Part model, mm, in its own coordinate system. Face numbers are marked on the shaded views. A direction names the side the tool comes from. Coordinates: 2 decimals unless noted, no trailing zeros. Write each loop counter-clockwise with the first axis right and the second up, starting at its lowest first coordinate (ties: lowest second). Pieces come first, ordered by that corner, then holes. Notation, with made-up numbers: (-9.75, 72.25) -> (27.25, 72.25) arc R15 cw to (27.25, 99.25) -> close; hole circle Ø5 at (7.25, -38.5). An arc over 180 degrees is marked (long way). One line per question, with ' | ' between items. Start each with the question number.
Item 1: Saw through at C-C (y = 12.5). List the corners of the cut face in (x, z).
Item 2: Probe probe 1 along Y at (x, z) = (0, 6.25); probe 2 along Y at (x, z) = (0.5, 2); probe 3 along X at (y, z) = (1, 11.5). List the from-to ranges inside material, lowest first. Write a range as [from, to].
Item 3: Saw through at A-A (x = 0). List the corners of the cut face in (y, z), and give its area (3 significant figures).
Item 4: Two-plate mould, pull along Y, no slides. Class the marked faces 1 and 2: pulls with the +Y half, pulls with the -Y half, needs draft (parallel to the pull), parting line crosses it, or undercut.
Item 5: Saw through at B-B (z = 6). Count the separate pieces of the cut face and the enclosed holes in it, and give its area (3 significant figures).
Item 6: 3-axis set-ups, long thin cutter, end or side, ignore diameter. For the marked faces 3 and 4: which of +Z, -Z, +X, -X, +Y, -Y reach the whole face in a straight line?
Item 7: Pin check, flat tips, straight feed: pin 1 (5 mm diameter, centred on x = 9.5, z = 2.5, fed in from -Y); pin 2 (13 mm diameter, centred on x = -40.7, y = 23.5, fed in from -Z); pin 3 (1.5 mm diameter, centred on x = -41, z = 14, fed in from +Y). Stop position of each tip, or through.
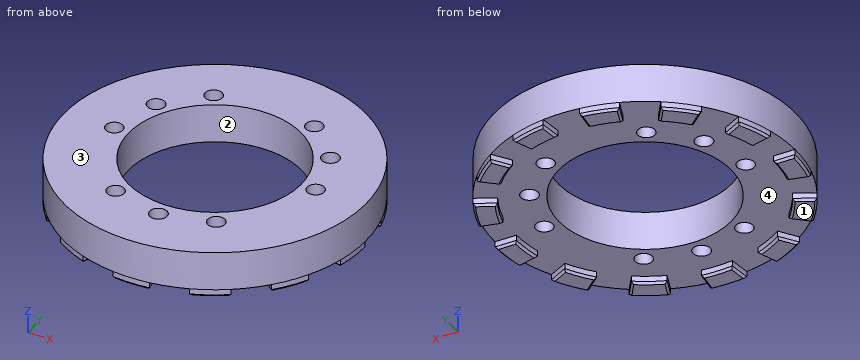
from build123d import *

# Parameters (mm, degrees)
SKETCH_1_R               = 70
SKETCH_1_R_2             = 40
EXTRUDE_1_DEPTH          = 18
SKETCH_2_R               = 4
CUT_EXTRUDE_1_DEPTH      = 20
PATTERN_CIRCULAR_1_COUNT = 6
SKETCH_3_R               = 4.06
CUT_EXTRUDE_2_DEPTH      = 20
PATTERN_CIRCULAR_2_COUNT = 3
EXTRUDE_2_DEPTH          = 3.5
CHAMFER_1_SIZE           = 1


with BuildPart() as part:
    # 草图1 → 凸台-拉伸1 (new body)
    with BuildSketch(Plane.XY):
        Circle(SKETCH_1_R)
        Circle(SKETCH_1_R_2, mode=Mode.SUBTRACT)
    extrude(amount=EXTRUDE_1_DEPTH)

    # 草图2 → 切除-拉伸1 (cut)
    with BuildSketch(Plane.XY.offset(18)):
        with Locations((47, 0)):
            Circle(SKETCH_2_R)
    cut_extrude_1 = extrude(amount=-CUT_EXTRUDE_1_DEPTH, mode=Mode.SUBTRACT)

    # 阵列(圆周)1: 切除-拉伸1 ×6 about axis
    pattern_circular_1_axis = Axis((0, 0, 0), (0, 0, 1))
    for i in range(1, PATTERN_CIRCULAR_1_COUNT):
        add(cut_extrude_1.rotate(pattern_circular_1_axis, i * 360 / PATTERN_CIRCULAR_1_COUNT), mode=Mode.SUBTRACT)

    # 草图3 → 切除-拉伸2 (cut)
    with BuildSketch(Plane.XY.offset(18)):
        with Locations((40.703193978, 23.5)):
            Circle(SKETCH_3_R)
    cut_extrude_2 = extrude(amount=-CUT_EXTRUDE_2_DEPTH, mode=Mode.SUBTRACT)

    # 阵列(圆周)2: 切除-拉伸2 ×3 about axis
    pattern_circular_2_axis = Axis((0, 0, 0), (0, 0, 1))
    for i in range(1, PATTERN_CIRCULAR_2_COUNT):
        add(cut_extrude_2.rotate(pattern_circular_2_axis, i * 360 / PATTERN_CIRCULAR_2_COUNT), mode=Mode.SUBTRACT)

    # 草图4 → 凸台-拉伸2 (add)
    with BuildSketch(Plane(origin=(0, 0, 0), x_dir=(-1, 0, 0), z_dir=(0, 0, -1))):
        with BuildLine():
            Line((60, 0), (70, 0))
            ThreePointArc((70, 0), (69.489621187, -8.437567618), (67.96592722, -16.7520965))
            Line((67.96592722, -16.7520965), (58.256509046, -14.358939857))
            ThreePointArc((58.256509046, -14.358939857), (59.562532446, -7.232200815), (60, 0))
        make_face()
        with BuildLine():
            Line((58.256509046, 14.358939857), (67.96592722, 16.7520965))
            ThreePointArc((67.96592722, 16.7520965), (65.451136988, 24.822342093), (61.981921796, 32.530622043))
            Line((61.981921796, 32.530622043), (53.127361539, 27.883390323))
            ThreePointArc((53.127361539, 27.883390323), (56.100974561, 21.276293223), (58.256509046, 14.358939857))
        make_face()
        with BuildLine():
            Line((44.91064489, 39.787359494), (52.395752372, 46.418586077))
            ThreePointArc((52.395752372, 46.418586077), (46.418586077, 52.395752372), (39.764532271, 57.608870613))
            Line((39.764532271, 57.608870613), (34.083884804, 49.379031954))
            ThreePointArc((34.083884804, 49.379031954), (39.787359494, 44.91064489), (44.91064489, 39.787359494))
        make_face()
        with BuildLine():
            Line((21.276293223, 56.100974561), (24.822342093, 65.451136988))
            ThreePointArc((24.822342093, 65.451136988), (16.7520965, 67.96592722), (8.437567618, 69.489621187))
            Line((8.437567618, 69.489621187), (7.232200815, 59.562532446))
            ThreePointArc((7.232200815, 59.562532446), (14.358939857, 58.256509046), (21.276293223, 56.100974561))
        make_face()
        with BuildLine():
            Line((-7.232200815, 59.562532446), (-8.437567618, 69.489621187))
            ThreePointArc((-8.437567618, 69.489621187), (-16.7520965, 67.96592722), (-24.822342093, 65.451136988))
            Line((-24.822342093, 65.451136988), (-21.276293223, 56.100974561))
            ThreePointArc((-21.276293223, 56.100974561), (-14.358939857, 58.256509046), (-7.232200815, 59.562532446))
        make_face()
        with BuildLine():
            Line((-34.083884804, 49.379031954), (-39.764532271, 57.608870613))
            ThreePointArc((-39.764532271, 57.608870613), (-46.418586077, 52.395752372), (-52.395752372, 46.418586077))
            Line((-52.395752372, 46.418586077), (-44.91064489, 39.787359494))
            ThreePointArc((-44.91064489, 39.787359494), (-39.787359494, 44.91064489), (-34.083884804, 49.379031954))
        make_face()
        with BuildLine():
            Line((-53.127361539, 27.883390323), (-61.981921796, 32.530622043))
            ThreePointArc((-61.981921796, 32.530622043), (-65.451136988, 24.822342093), (-67.96592722, 16.7520965))
            Line((-67.96592722, 16.7520965), (-58.256509046, 14.358939857))
            ThreePointArc((-58.256509046, 14.358939857), (-56.100974561, 21.276293223), (-53.127361539, 27.883390323))
        make_face()
        with BuildLine():
            Line((-60, 0), (-70, 0))
            ThreePointArc((-70, 0), (-69.489621187, -8.437567618), (-67.96592722, -16.7520965))
            Line((-67.96592722, -16.7520965), (-58.256509046, -14.358939857))
            ThreePointArc((-58.256509046, -14.358939857), (-59.562532446, -7.232200815), (-60, 0))
        make_face()
        with BuildLine():
            Line((-53.127361539, -27.883390323), (-61.981921796, -32.530622043))
            ThreePointArc((-61.981921796, -32.530622043), (-57.608870613, -39.764532271), (-52.395752372, -46.418586077))
            Line((-52.395752372, -46.418586077), (-44.91064489, -39.787359494))
            ThreePointArc((-44.91064489, -39.787359494), (-49.379031954, -34.083884804), (-53.127361539, -27.883390323))
        make_face()
        with BuildLine():
            Line((-34.083884804, -49.379031954), (-39.764532271, -57.608870613))
            ThreePointArc((-39.764532271, -57.608870613), (-32.530622043, -61.981921796), (-24.822342093, -65.451136988))
            Line((-24.822342093, -65.451136988), (-21.276293223, -56.100974561))
            ThreePointArc((-21.276293223, -56.100974561), (-27.883390323, -53.127361539), (-34.083884804, -49.379031954))
        make_face()
        with BuildLine():
            Line((-7.232200815, -59.562532446), (-8.437567618, -69.489621187))
            ThreePointArc((-8.437567618, -69.489621187), (0, -70), (8.437567618, -69.489621187))
            Line((8.437567618, -69.489621187), (7.232200815, -59.562532446))
            ThreePointArc((7.232200815, -59.562532446), (0, -60), (-7.232200815, -59.562532446))
        make_face()
        with BuildLine():
            Line((21.276293223, -56.100974561), (24.822342093, -65.451136988))
            ThreePointArc((24.822342093, -65.451136988), (32.530622043, -61.981921796), (39.764532271, -57.608870613))
            Line((39.764532271, -57.608870613), (34.083884804, -49.379031954))
            ThreePointArc((34.083884804, -49.379031954), (27.883390323, -53.127361539), (21.276293223, -56.100974561))
        make_face()
        with BuildLine():
            Line((44.91064489, -39.787359494), (52.395752372, -46.418586077))
            ThreePointArc((52.395752372, -46.418586077), (57.608870613, -39.764532271), (61.981921796, -32.530622043))
            Line((61.981921796, -32.530622043), (53.127361539, -27.883390323))
            ThreePointArc((53.127361539, -27.883390323), (49.379031954, -34.083884804), (44.91064489, -39.787359494))
        make_face()
    extrude(amount=EXTRUDE_2_DEPTH)

    # 倒角1
    chamfer_1_edges = [part.edges().sort_by_distance(p)[0] for p in [
        (-23.049317658, -60.776055775, -3.5),
        (-27.883390323, -53.127361539, -3.5),
        (-36.924208538, -53.493951283, -3.5),
        (-32.530622043, -61.981921796, -3.5),
        (7.834884217, -64.526076816, -3.5),
        (0, -60, -3.5),
        (-7.834884217, -64.526076816, -3.5),
        (0, -70, -3.5),
        (36.924208538, -53.493951283, -3.5),
        (27.883390323, -53.127361539, -3.5),
        (23.049317658, -60.776055775, -3.5),
        (32.530622043, -61.981921796, -3.5),
        (57.554641667, -30.207006183, -3.5),
        (49.379031954, -34.083884804, -3.5),
        (48.653198631, -43.102972786, -3.5),
        (57.608870613, -39.764532271, -3.5),
        (65, 0, -3.5),
        (59.562532446, -7.232200815, -3.5),
        (63.111218133, -15.555518179, -3.5),
        (69.489621187, -8.437567618, -3.5),
        (57.554641667, 30.207006183, -3.5),
        (56.100974561, 21.276293223, -3.5),
        (63.111218133, 15.555518179, -3.5),
        (65.451136988, 24.822342093, -3.5),
        (36.924208538, 53.493951283, -3.5),
        (39.787359494, 44.91064489, -3.5),
        (48.653198631, 43.102972786, -3.5),
        (46.418586077, 52.395752372, -3.5),
        (7.834884217, 64.526076816, -3.5),
        (14.358939857, 58.256509046, -3.5),
        (23.049317658, 60.776055775, -3.5),
        (16.7520965, 67.96592722, -3.5),
        (-23.049317658, 60.776055775, -3.5),
        (-14.358939857, 58.256509046, -3.5),
        (-7.834884217, 64.526076816, -3.5),
        (-16.7520965, 67.96592722, -3.5),
        (-48.653198631, 43.102972786, -3.5),
        (-39.787359494, 44.91064489, -3.5),
        (-36.924208538, 53.493951283, -3.5),
        (-46.418586077, 52.395752372, -3.5),
        (-63.111218133, 15.555518179, -3.5),
        (-56.100974561, 21.276293223, -3.5),
        (-57.554641667, 30.207006183, -3.5),
        (-65.451136988, 24.822342093, -3.5),
        (-63.111218133, -15.555518179, -3.5),
        (-59.562532446, -7.232200815, -3.5),
        (-65, 0, -3.5),
        (-69.489621187, -8.437567618, -3.5),
        (-48.653198631, -43.102972786, -3.5),
        (-49.379031954, -34.083884804, -3.5),
        (-57.554641667, -30.207006183, -3.5),
        (-57.608870613, -39.764532271, -3.5),
    ]]
    chamfer(chamfer_1_edges, length=CHAMFER_1_SIZE)


solid = part.part
From the geometry:
1) outline: (-68.87, 0) -> (-38, 0) -> (-38, 18) -> (-68.87, 18) -> close; (38, 0) -> (68.87, 0) -> (68.87, 18) -> (38, 18) -> close
2) probe 1: [-70, -51.06], [-42.94, -40], [40, 70] | probe 2: [-70, -51.03], [-42.97, -40], [40, 70] | probe 3: [-69.99, -50.87], [-43.13, -39.99], [39.99, 43.13], [50.87, 69.99]
3) outline: (-70, -2.5) -> (-69, -3.5) -> (-61, -3.5) -> (-60, -2.5) -> (-60, 0) -> (-51.06, 0) -> (-51.06, 18) -> (-70, 18) -> close; (-42.94, 0) -> (-40, 0) -> (-40, 18) -> (-42.94, 18) -> close; (40, 0) -> (70, 0) -> (70, 18) -> (40, 18) -> close | area: 968 mm2
4) face 1: needs draft | face 2: undercut
5) separate pieces: 1 | enclosed holes: 10 | area: 9,910 mm2
6) face 3: +Z, +X, -X, +Y, -Y | face 4: -Z
7) pin 1: y = -69.65 | pin 2: z = 0 | pin 3: y = 57.27
